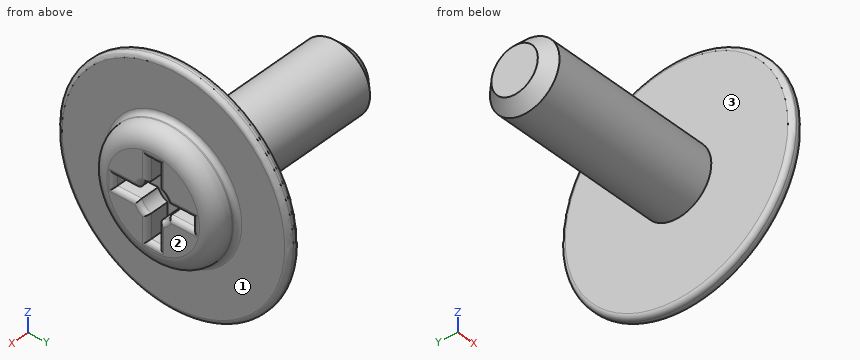
```python
from build123d import *

# Parameters (mm, degrees)
ESQUISSE2_W                  = 0.5
ESQUISSE2_H                  = 1.7
ENL_V_MAT_EXTRU_1_DEPTH      = 1
R_P_TITION_CIRCULAIRE1_COUNT = 4
ESQUISSE3_R                  = 0.699771755
ENL_V_MAT_EXTRU_2_DEPTH      = 1
CHANFREIN1_SIZE              = 0.5
CONG_1_R                     = 0.2


with BuildPart() as part:
    # Esquisse1 → Révolution1 (revolve)
    with BuildSketch(Plane.XY, mode=Mode.PRIVATE) as r_volution1_sk:
        with BuildLine():
            Line((0, 0), (0, 1.5))
            Line((0, 1.5), (8, 1.5))
            Line((8, 1.5), (8, 5))
            Line((8, 5), (8.5, 5))
            Line((8.5, 5), (8.5, 2.75))
            Line((8.5, 2.75), (8.75, 2.75))
            ThreePointArc((8.75, 2.75), (9.280330086, 2.530330086), (9.5, 2))
            Line((9.5, 2), (9.5, 0))
            Line((9.5, 0), (0, 0))
        make_face()
    revolve(r_volution1_sk.sketch.rotate(Axis((0, 0, 0), (1, 0, 0)), 90), axis=Axis((0, 0, 0), (1, 0, 0)))

    # Esquisse2 → Enlèv. mat.-Extru.1 (cut)
    with BuildSketch(Plane(origin=(9.5, 0, 0), x_dir=(0, 0, -1), z_dir=(1, 0, 0))):
        with Locations((0, 0.85)):
            Rectangle(ESQUISSE2_W, ESQUISSE2_H)
    enl_v_mat_extru_1 = extrude(amount=-ENL_V_MAT_EXTRU_1_DEPTH, mode=Mode.SUBTRACT)

    # Répétition circulaire1: Enlèv. mat.-Extru.1 ×4 about axis
    r_p_tition_circulaire1_axis = Axis((0, 0, 0), (1, 0, 0))
    for i in range(1, R_P_TITION_CIRCULAIRE1_COUNT):
        add(enl_v_mat_extru_1.rotate(r_p_tition_circulaire1_axis, i * 360 / R_P_TITION_CIRCULAIRE1_COUNT), mode=Mode.SUBTRACT)

    # Esquisse3 → Enlèv. mat.-Extru.2 (cut)
    with BuildSketch(Plane(origin=(9.5, 0, 0), x_dir=(0, 0, -1), z_dir=(1, 0, 0))):
        Circle(ESQUISSE3_R)
    extrude(amount=-ENL_V_MAT_EXTRU_2_DEPTH, mode=Mode.SUBTRACT)

    # Chanfrein1
    chanfrein1_edges = [part.edges().sort_by_distance(p)[0] for p in [
        (0, 0, -1.5),
    ]]
    chamfer(chanfrein1_edges, length=CHANFREIN1_SIZE)

    # Congé1
    cong_1_edges = [part.edges().sort_by_distance(p)[0] for p in [
        (8, 0, -5),
        (8.5, 0, -5),
        (8.5, 0, -2.75),
        (9.5, 0, 1.7),
        (9.5, -0.25, 1.176795238),
        (9.5, -0.494813353, 0.494813353),
        (9.5, -1.176795238, 0.25),
        (9.5, -1.7, 0),
        (9.5, -1.176795238, -0.25),
        (9.5, -0.494813353, -0.494813353),
        (9.5, -0.25, -1.176795238),
        (9.5, 0, -1.7),
        (9.5, 0.25, -1.176795238),
        (9.5, 0.494813353, -0.494813353),
        (9.5, 1.176795238, -0.25),
        (9.5, 1.7, 0),
        (9.5, 1.176795238, 0.25),
        (9.5, 0.494813353, 0.494813353),
        (9.5, 0.25, 1.176795238),
    ]]
    fillet(cong_1_edges, radius=CONG_1_R)


solid = part.part
```
Model file for the job. Use its own axes, mm. Face numbers are marked on the shaded views. A direction names the side the tool comes from. Give positions to 0.01 mm unless a question says otherwise; leave off trailing zeros. Order: outer loops, then holes, each group sorted by start corner. A loop starts at its lowest first (then second) coordinate and runs counter-clockwise, first axis right, second up.
1) Saw through at A-A, the plane z = 0. Write the cut outline in (x, y).
2) Saw through at C-C, the plane x = 1.75. Write the cut outline in (y, z).
3) Wall check: probe 1 along X at (y, z) = (0.25, 2); probe 2 along X at (y, z) = (3, -0.25); probe 3 along Y at (x, z) = (9, -1.25). Give the ranges that are in metal, low to high.
4) 3-axis set-ups, long thin cutter, end or side, ignore diameter. For the marked faces 1, 2 and 3: which of +Z, -Z, +X, -X, +Y, -Y reach the whole face in a straight line?
5) Pin check, flat tips, straight feed: pin 1 (2 mm diameter, centred on x = 1.5, z = -1.5, fed in from +Y); pin 2 (0.6 mm diameter, centred on x = 9, y = 0, fed in from +Z); pin 3 (3 mm diameter, centred on x = 5, y = 2, fed in from -Z). Stop position of each tip, or through.
Computed:
1. outline: (0, -1) - (0.5, -1.5) - (8, -1.5) - (8, -4.8) arc R0.2 ccw to (8.2, -5) - (8.3, -5) arc R0.2 ccw to (8.5, -4.8) - (8.5, -2.95) arc R0.2 cw to (8.7, -2.75) - (8.75, -2.75) arc R0.75 ccw to (9.5, -2) - (9.5, -1.9) arc R0.2 ccw to (9.3, -1.7) - (8.5, -1.7) - (8.5, 1.7) - (9.3, 1.7) arc R0.2 ccw to (9.5, 1.9) - (9.5, 2) arc R0.75 ccw to (8.75, 2.75) - (8.7, 2.75) arc R0.2 cw to (8.5, 2.95) - (8.5, 4.8) arc R0.2 ccw to (8.3, 5) - (8.2, 5) arc R0.2 ccw to (8, 4.8) - (8, 1.5) - (0.5, 1.5) - (0, 1) - close
2. outline: circle Ø3 at (0, 0)
3. probe 1: x = 8 to 9.5
3. probe 2: x = 8 to 8.5
3. probe 3: y = -2.4 to -0.25, 0.25 to 2.4
4. face 1: +X
4. face 2: +Z, -Z, +X, +Y, -Y
4. face 3: -X
5. pin 1: stops at y = 1.41
5. pin 2: stops at z = 2.75
5. pin 3: stops at z = -1.41
